Geometry check sheet. Reference: the model listing, model coordinates, mm. A direction names the side the tool comes from. Round coordinates to 2 decimals unless told otherwise and drop trailing zeros. Order: outer loops, then holes, each group sorted by start corner. A loop starts at its lowest first (then second) coordinate and runs counter-clockwise, first axis right, second up. Notation, with made-up numbers: (51, 85.5) -> (98, 85.5) arc R20 cw to (98, 93.5) -> close; hole circle Ø9 at (21.25, -15). An arc over 180 degrees is marked (long way). Use a Markdown table: item, result. Add a question column.
Item 1: Set-up check for faces 1 (the flat face through (33, 1, 14.5)), 2 (the flat face through (21, 0, 12)), 3 (the flat face through (29.785, 4, 12)): record each of +Z, -Z, +X, -X, +Y, -Y from which the full face is reachable in a straight line by a thin tool's end or side.
Item 2: Sectioned sample at A-A, the plane x = 30.5. Record the cut outline in (y, z).
Item 3: Mould release check, pull along Z, two halves, no side actions. Record for faces 4 (the flat face through (0, 31, 12)), 5 (the flat face through (21, 32, 25)), 6 (the flat face through (33, 5, 12)): pulls with the +Z half, pulls with the -Z half, needs draft (parallel to the pull), parting line crosses it, or undercut.
Item 4: Sectioned sample at B-B, the plane z = 16.75. Record the cut outline in (x, y) (3 decimals).
Item 5: Material ranges on probe 1 along Y at (x, z) = (35.5, 10.25), recorded low to high. Write a range as [from, to].
from build123d import *

# Parameters (mm, degrees)
SKETCH1_W           = 43.57
SKETCH1_H           = 63.5
BOSS_EXTRUDE1_DEPTH = 25
CUT_EXTRUDE2_DEPTH  = 81.966628311
SKETCH4_W           = 43.57
SKETCH4_H           = 25
SKETCH4_W_2         = 6
SKETCH4_H_2         = 15
BOSS_EXTRUDE2_DEPTH = 9


with BuildPart() as part:
    # Sketch1 → Boss-Extrude1 (new body)
    with BuildSketch(Plane.XY):
        with Locations((21.785, 31.75)):
            Rectangle(SKETCH1_W, SKETCH1_H)
    extrude(amount=BOSS_EXTRUDE1_DEPTH)

    # Sketch3 → Cut-Extrude2 (cut, through all)
    with BuildSketch(Plane(origin=(43.57, 0, 0), x_dir=(0, 0, -1), z_dir=(1, 0, 0))):
        with BuildLine():
            Line((-14.5, 0), (-14.5, 1.5))
            ThreePointArc((-14.5, 1.5), (-14.060660172, 2.560660172), (-13, 3))
            Line((-13, 3), (-12, 3))
            ThreePointArc((-12, 3), (-10.939339828, 2.560660172), (-10.5, 1.5))
            Line((-10.5, 1.5), (-10.5, 0))
            Line((-10.5, 0), (-7.5, 0))
            Line((-7.5, 0), (-7.5, 3.5))
            ThreePointArc((-7.5, 3.5), (-7.939339828, 4.560660172), (-9, 5))
            Line((-9, 5), (-16, 5))
            ThreePointArc((-16, 5), (-17.060660172, 4.560660172), (-17.5, 3.5))
            Line((-17.5, 3.5), (-17.5, 0))
            Line((-17.5, 0), (-14.5, 0))
        make_face()
    extrude(amount=-CUT_EXTRUDE2_DEPTH, mode=Mode.SUBTRACT)


with BuildPart() as cut_extrude2_piece_1:
    # of the separate pieces the step leaves, piece 1, a body of its own (cut_extrude2_pieces)
    add(part.part.solids().sort_by_distance((0, 0, 0))[0])



with BuildPart() as cut_extrude2_piece_2:
    # of the separate pieces the step leaves, piece 2, a body of its own (cut_extrude2_pieces)
    add(part.part.solids().sort_by_distance((43.57, 0, 10.5))[0])


with BuildPart() as cut_extrude2_piece_1_1:
    add(cut_extrude2_piece_1.part)

    add(cut_extrude2_piece_2.part)  # Boss-Extrude2 merges Cut-Extrude2 piece 2
    # Sketch4 → Boss-Extrude2 (add)
    with BuildSketch(Plane.XZ):
        with Locations((21.785, 12.5)):
            Rectangle(SKETCH4_W, SKETCH4_H)
        with Locations((10.785, 12.5)):
            Rectangle(SKETCH4_W_2, SKETCH4_H_2, mode=Mode.SUBTRACT)
        with Locations((32.785, 12.5)):
            Rectangle(SKETCH4_W_2, SKETCH4_H_2, mode=Mode.SUBTRACT)
    extrude(amount=-BOSS_EXTRUDE2_DEPTH)


solid = cut_extrude2_piece_1_1.part
Found:
| question | item | result |
|---|---|---|
| 1 | face 1 | -Y |
| 1 | face 2 | +Z, -Z, +X, -X, -Y |
| 1 | face 3 | none |
| 2 | outline | (0, 0) -> (63.5, 0) -> (63.5, 25) -> (0, 25) -> (0, 17.5) -> (3.5, 17.5) arc R1.5 cw to (5, 16) -> (5, 9) arc R1.5 cw to (3.5, 7.5) -> (0, 7.5) -> close; (0, 10.5) -> (1.5, 10.5) arc R1.5 ccw to (3, 12) -> (3, 13) arc R1.5 ccw to (1.5, 14.5) -> (0, 14.5) -> close |
| 3 | face 4 | needs draft |
| 3 | face 5 | pulls with the +Z half |
| 3 | face 6 | undercut |
| 4 | outline | (0, 0) -> (7.785, 0) -> (7.785, 4.799) -> (13.785, 4.799) -> (13.785, 0) -> (29.785, 0) -> (29.785, 4.799) -> (35.785, 4.799) -> (35.785, 0) -> (43.57, 0) -> (43.57, 63.5) -> (0, 63.5) -> close |
| 5 | probe 1 | y = [5, 63.5] |
